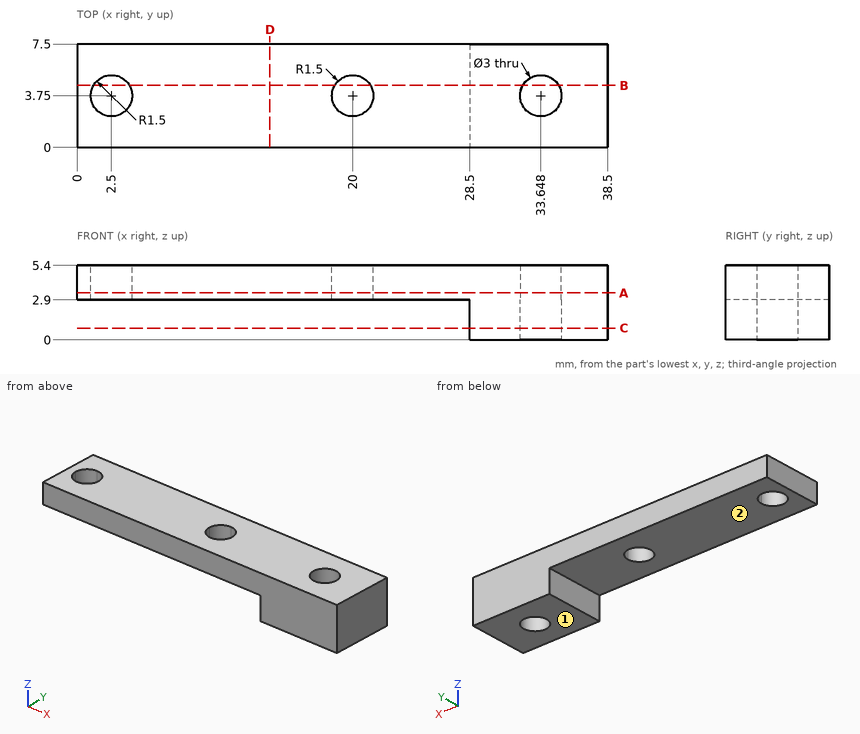
Can you work these out from the drawing? Everything is in mm from the part's minimum corner. A direction names the side the tool comes from. Round coordinates to 2 decimals unless told otherwise and drop trailing zeros. Order: outer loops, then holes, each group sorted by start corner. A loop starts at its lowest first (then second) coordinate and runs counter-clockwise, first axis right, second up. Notation, with made-up numbers: (9.25, 26.25) -> (37.25, 26.25) arc R22 cw to (37.25, 54.25) -> close; hole circle Ø10 at (71.25, 60.5). An arc over 180 degrees is marked (long way). Use CSV: the item, a comma, the result in double quotes.
1. I want a section at A-A on z = 3.4. List the corners of the cut face in (x, y) for me, and give its area (3 significant figures).
Recorded:
outline,"(0, 0) -> (38.5, 0) -> (38.5, 7.5) -> (0, 7.5) -> close; hole circle Ø3 at (2.5, 3.75); hole circle Ø3 at (20, 3.75); hole circle Ø3 at (33.65, 3.75)"
area,"268 mm2"
2. I want a section at B-B on y = 4.5. List the corners of the cut face in (x, z) for me.
Recorded:
outline,"(0, 2.9) -> (1.2, 2.9) -> (1.2, 5.4) -> (0, 5.4) -> close; (3.8, 2.9) -> (18.7, 2.9) -> (18.7, 5.4) -> (3.8, 5.4) -> close; (21.3, 2.9) -> (28.5, 2.9) -> (28.5, 0) -> (32.35, 0) -> (32.35, 5.4) -> (21.3, 5.4) -> close; (34.95, 0) -> (38.5, 0) -> (38.5, 5.4) -> (34.95, 5.4) -> close"
3. I want a section at D-D on x = 14. List the corners of the cut face in (y, z) for me.
Recorded:
outline,"(0, 2.9) -> (7.5, 2.9) -> (7.5, 5.4) -> (0, 5.4) -> close"
4. I want a section at C-C on z = 0.85. List the corners of the cut face in (x, y) for me.
Recorded:
outline,"(28.5, 0) -> (38.5, 0) -> (38.5, 7.5) -> (28.5, 7.5) -> close; hole circle Ø3 at (33.65, 3.75)"
5. I'm going to push flat-ended pins straight in: P1, Ø0.9, axis at y = 4, z = 1, coming from the -X side; P2, Ø1, axis at x = 16.5, y = 2.5, coming from the -Z side. Where does each tip first touch, or does it pass through?
Recorded:
P1,"stops at x = 28.5"
P2,"stops at z = 2.9"
6. Which directions (+Z, -Z, +X, -X, +Y, -Y) give clear straight access to the entire face, cutting with the end or side of a thin tool? Please do the marked faces 1 and 2.
Recorded:
face 1,"-Z, +X, -X, +Y, -Y"
face 2,"-Z, -X, +Y, -Y"
7. I need wall thicknesses on line 1 along X through (y, z) = (3.75, 2.1); line 2 along X through (y, z) = (3.75, 4.25); line 3 along X through (y, z) = (4, 3.15). Which ranges of each line are inside material? Lowest first, please.
Recorded:
line 1,"x = 28.5 to 32.15, 35.15 to 38.5"
line 2,"x = 0 to 1, 4 to 18.5, 21.5 to 32.15, 35.15 to 38.5"
line 3,"x = 0 to 1.02, 3.98 to 18.52, 21.48 to 32.17, 35.13 to 38.5"
